Geometry: final body of the model. Coordinates: model frame, mm. A direction names the side the tool comes from. Coordinates: 2 decimals unless noted, no trailing zeros. Order: outer loops, then holes, each group sorted by start corner. A loop starts at its lowest first (then second) coordinate and runs counter-clockwise, first axis right, second up. Notation, with made-up numbers: (32, 28) - (49, 28) arc R5 cw to (49, 36) - close; hole circle Ø5 at (56, -32). An arc over 180 degrees is marked (long way). Use a Markdown table: item, result. Add a question column.
```python
from build123d import *

# Parameters (mm, degrees)
F0_R     = 238
F0_R_2   = 235.5
F1_DEPTH = 460
F2_R     = 238
F3_DEPTH = 5
F5_D     = 250
F5_DEPTH = 430


with BuildPart() as f1:
    # F0 (on Right) → F1 (new body)
    with BuildSketch(Plane.YZ):
        Circle(F0_R)
        Circle(F0_R_2, mode=Mode.SUBTRACT)
    extrude(amount=F1_DEPTH)

    # F2 (on Right) → F3 (join)
    with BuildSketch(Plane.YZ):
        Circle(F2_R)
    extrude(amount=F3_DEPTH)

    # F5
    with Locations(Plane(origin=(0, 0, 0), x_dir=(0, -1, 0), z_dir=(-1, 0, 0))):
        with Locations((0, 0)):
            Hole(F5_D / 2, depth=F5_DEPTH)


solid = f1.part
```
1) Set-up query: faces 1 (the face through (2.54, -124.88, 5.5)), 2 (the face through (5, 101, -101)). Return all of +Z, -Z, +X, -X, +Y, -Y with unobstructed straight access to the full face (end or side cutting, diameter ignored); none if empty.
2) Pin query (flat end, axial travel): pin 1 (3 mm diameter, centred on x = 217, y = -94, fed in from -Z); pin 2 (12 mm diameter, centred on x = 327, z = -127.5, fed in from -Y); pin 3 (12 mm diameter, centred on y = 66.5, z = 121, fed in from +X); pin 4 (10 mm diameter, centred on y = -148, z = 57.5, fed in from -X). Return the tip coordinate at first contact, or that it passes through.
3) Section A-A (z = 0). Return loops of the section in (x, y), then the cut area to 4 significant figures.
4) Section C-C (x = 147). Return loops of the section in (y, z).
5) Section D-D (z = 193). Return loops of the section in (x, y).
6) Draft query along Y for faces 3 (the face through (226.78, 127.95, 200.68)), 4 (the face through (229.315, -173.573, 159.162)), 5 (the face through (0, 102, -102)). Return one class per face: pulls with the +Y half, pulls with the -Y half, needs draft (parallel to the pull), parting line crosses it, or undercut.
7) Ray query, line 1 along Z through (x, y) = (417.5, -2.5); line 2 along Z through (x, y) = (3, 0); line 3 along X through (y, z) = (-125, 109). Return the intervals inside material, ascending.
Values follow:
| question | item | result |
|---|---|---|
| 1 | face 1 | +X, -X |
| 1 | face 2 | +X |
| 2 | pin 1 | stops at z = -219.29 |
| 2 | pin 2 | stops at y = -204.65 |
| 2 | pin 3 | stops at x = 5 |
| 2 | pin 4 | stops at x = 0 |
| 3 | outline | (0, -238) - (460, -238) - (460, -235.5) - (5, -235.5) - (5, -125) - (0, -125) - close; (0, 125) - (5, 125) - (5, 235.5) - (460, 235.5) - (460, 238) - (0, 238) - close |
| 3 | area | 3,405 mm² |
| 4 | outline | circle Ø476 at (0, 0); hole circle Ø471 at (0, 0) |
| 5 | outline | (0, -139.27) - (460, -139.27) - (460, -134.95) - (5, -134.95) - (5, 134.95) - (460, 134.95) - (460, 139.27) - (0, 139.27) - close |
| 6 | face 3 | parting line crosses it |
| 6 | face 4 | undercut |
| 6 | face 5 | needs draft |
| 7 | line 1 | z = -237.99 to -235.49, 235.49 to 237.99 |
| 7 | line 2 | z = -238 to -125, 125 to 238 |
| 7 | line 3 | x = 0 to 5 |
